The listing builds one solid part. Answer for the finished solid, in the listing's coordinates (mm). Face numbers are marked on the shaded views. A direction names the side the tool comes from. Round coordinates to 2 decimals unless told otherwise and drop trailing zeros. Loops run counter-clockwise (first coordinate to the right, second up) from the corner with the lowest first, then second, coordinate; pieces in that order, holes last. Notation, with made-up numbers: (77, 17.5) -> (82, 17.5) arc R24 ccw to (82, 28.5) -> close; hole circle Ø2 at (29.5, 87.25). An arc over 180 degrees is marked (long way). Use a Markdown table: item, result. Add a question column.
Q1. Consider line 1 (Y direction, x = 0, z = 29); line 2 (Z direction, x = 0, y = -13); line 3 (Z direction, x = 4, y = -4). Determine where each line is inside the solid, lowest interval first.
Q2. Section C-C on z = 66 is taken. Give the vertices of the cut face in (x, y).
Q3. Section B-B on y = 0 is taken. Give the vertices of the cut face in (x, z).
Q4. Section A-A on x = 0 is taken. Give the vertices of the cut face in (y, z).
Q5. Which of the six approach directions +Z, -Z, +X, -X, +Y, -Y give full straight-line access (tool end or side, diameter ignored) to the marked faces 1, 2 and 3?
Q6. Section D-D on y = 17.5 is taken. Give the vertices of the cut face in (x, z), then the cut area to 3 significant figures.
Q7. Given pin 1 Ø5 at (x, y) = (-17.5, 0) entering from -Z; pin 2 Ø1 at (y, z) = (-3, 44) entering from -X; pin 3 Ø6.5 at (x, y) = (17.5, 0) entering from +Z, each flat-ended and moving along its own axis, determine where each tip first touches the part or whether it passes through.
from build123d import *

# Parameters (mm, degrees)
SKETCH1_R           = 24.75
BOSS_EXTRUDE1_DEPTH = 31
SKETCH2_R           = 3
BOSS_EXTRUDE2_DEPTH = 44
SKETCH6_R           = 2
CUT_EXTRUDE3_DEPTH  = 5
CIRPATTERN1_COUNT   = 4
SKETCH5_R           = 2
CUT_EXTRUDE2_DEPTH  = 10
CIRPATTERN2_COUNT   = 2
SKETCH7_R           = 9
BOSS_EXTRUDE3_DEPTH = 7


with BuildPart() as part:
    # Sketch1 → Boss-Extrude1 (new body, symmetric)
    with BuildSketch(Plane.XY):
        Circle(SKETCH1_R)
    extrude(amount=BOSS_EXTRUDE1_DEPTH, both=True)

    # Sketch2 → Boss-Extrude2 (add)
    with BuildSketch(Plane.XY.offset(31)):
        Circle(SKETCH2_R)
    extrude(amount=BOSS_EXTRUDE2_DEPTH)

    # Sketch6 → Cut-Extrude3 (cut)
    with BuildSketch(Plane.XY.offset(31)):
        with Locations((0, 17.5)):
            Circle(SKETCH6_R)
    cut_extrude3 = extrude(amount=-CUT_EXTRUDE3_DEPTH, mode=Mode.SUBTRACT)

    # CirPattern1: Cut-Extrude3 ×4 about axis
    cirpattern1_axis = Axis((0, 0, 0), (0, 0, 1))
    for i in range(1, CIRPATTERN1_COUNT):
        add(cut_extrude3.rotate(cirpattern1_axis, i * 360 / CIRPATTERN1_COUNT), mode=Mode.SUBTRACT)

    # Sketch5 → Cut-Extrude2 (cut)
    with BuildSketch(Plane(origin=(0, 0, -31), x_dir=(-1, 0, 0), z_dir=(0, 0, -1))):
        with Locations((-17.5, 0)):
            Circle(SKETCH5_R)
    cut_extrude2 = extrude(amount=-CUT_EXTRUDE2_DEPTH, mode=Mode.SUBTRACT)

    # CirPattern2: Cut-Extrude2 ×2 about axis
    cirpattern2_axis = Axis((0, 0, 0), (0, 0, 1))
    for i in range(1, CIRPATTERN2_COUNT):
        add(cut_extrude2.rotate(cirpattern2_axis, i * 360 / CIRPATTERN2_COUNT), mode=Mode.SUBTRACT)

    # Sketch7 → Boss-Extrude3 (add)
    with BuildSketch(Plane(origin=(0, 0, -31), x_dir=(-1, 0, 0), z_dir=(0, 0, -1))):
        Circle(SKETCH7_R)
    extrude(amount=BOSS_EXTRUDE3_DEPTH)


solid = part.part
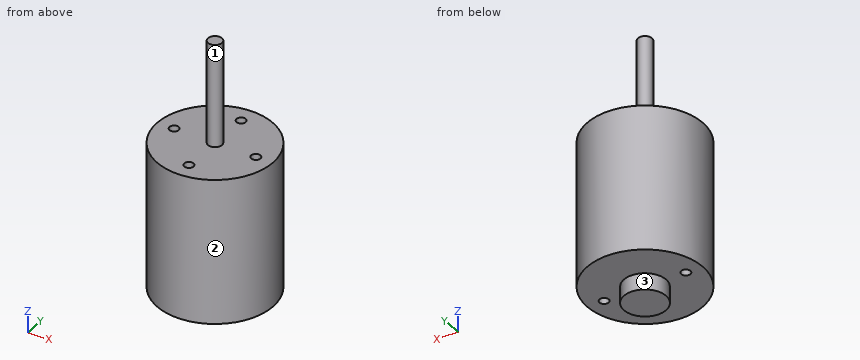
Checked values:
| question | item | result |
|---|---|---|
| 1 | line 1 | y = -24.75 to -19.5, -15.5 to 15.5, 19.5 to 24.75 |
| 1 | line 2 | z = -31 to 31 |
| 1 | line 3 | z = -38 to 31 |
| 2 | outline | circle Ø6 at (0, 0) |
| 3 | outline | (-24.75, -31) -> (-19.5, -31) -> (-19.5, -21) -> (-15.5, -21) -> (-15.5, -31) -> (-9, -31) -> (-9, -38) -> (9, -38) -> (9, -31) -> (15.5, -31) -> (15.5, -21) -> (19.5, -21) -> (19.5, -31) -> (24.75, -31) -> (24.75, 31) -> (19.5, 31) -> (19.5, 26) -> (15.5, 26) -> (15.5, 31) -> (3, 31) -> (3, 75) -> (-3, 75) -> (-3, 31) -> (-15.5, 31) -> (-15.5, 26) -> (-19.5, 26) -> (-19.5, 31) -> (-24.75, 31) -> close |
| 4 | outline | (-24.75, -31) -> (-9, -31) -> (-9, -38) -> (9, -38) -> (9, -31) -> (24.75, -31) -> (24.75, 31) -> (19.5, 31) -> (19.5, 26) -> (15.5, 26) -> (15.5, 31) -> (3, 31) -> (3, 75) -> (-3, 75) -> (-3, 31) -> (-15.5, 31) -> (-15.5, 26) -> (-19.5, 26) -> (-19.5, 31) -> (-24.75, 31) -> close |
| 5 | face 1 | +Z |
| 5 | face 2 | +Z, -Z |
| 5 | face 3 | -Z |
| 6 | outline | (-17.5, -31) -> (17.5, -31) -> (17.5, 31) -> (2, 31) -> (2, 26) -> (-2, 26) -> (-2, 31) -> (-17.5, 31) -> close |
| 6 | area | 2,150 mm2 |
| 7 | pin 1 | stops at z = -31 |
| 7 | pin 2 | stops at x = -1.66 |
| 7 | pin 3 | stops at z = 31 |
